CAD build for the part. Positions are in the model's coordinates, mm. Round coordinates to 2 decimals unless told otherwise and drop trailing zeros. One line per question, with ' | ' between items.
```python
from build123d import *

# Parameters (mm, degrees)
SKETCH1_W           = 47.625
SKETCH1_H           = 47.625
SKETCH1_R           = 1.5875
BOSS_EXTRUDE1_DEPTH = 1.5875
FILLET1_R           = 4.7625


with BuildPart() as part:
    # Sketch1 → Boss-Extrude1 (new body)
    with BuildSketch(Plane(origin=(0, 0, 0), x_dir=(1, 0, 0), z_dir=(0, 1, 0))):
        Rectangle(SKETCH1_W, SKETCH1_H)
        with Locations((-19.05, 19.05)):
            Circle(SKETCH1_R, mode=Mode.SUBTRACT)
        with Locations((19.05, 19.05)):
            Circle(SKETCH1_R, mode=Mode.SUBTRACT)
        with Locations((19.05, -19.05)):
            Circle(SKETCH1_R, mode=Mode.SUBTRACT)
        with Locations((-19.05, -19.05)):
            Circle(SKETCH1_R, mode=Mode.SUBTRACT)
    extrude(amount=BOSS_EXTRUDE1_DEPTH)

    # Fillet1
    fillet1_edges = [part.edges().sort_by_distance(p)[0] for p in [
        (-23.8125, 0.79375, -23.8125),
        (23.8125, 0.79375, -23.8125),
        (23.8125, 0.79375, 23.8125),
        (-23.8125, 0.79375, 23.8125),
    ]]
    fillet(fillet1_edges, radius=FILLET1_R)


solid = part.part
```
(1) Two-plate mould, pull along X, no slides. Class faces 1 (the face through (-23.812, 1, 0)), 2 (the face through (-20.22, 0.783, 17.977)), 3 (the face through (0, 1, -23.812)), 4 (the face through (17.88, 0.783, 17.977)): released by +X, released by -X, zero draft, split by the parting line, or undercut.
Results found:
face 1: released by -X | face 2: undercut | face 3: zero draft | face 4: undercut
(2) Probe L1, parallel to Z at x = 19.05, y = 1.15; L2, parallel to Z at x = -21, y = 0.85. List the from-to ranges inside material, lowest first.
Results found:
L1: z = -23.81 to -20.64, -17.46 to 17.46, 20.64 to 23.81 | L2: z = -23.39 to 23.39
(3) Cut at A-A, the plane y = 0.5. State how many separate pieces and enclosed holes the cut face has, then the cut area to 3 significant figures.
Results found:
separate pieces: 1 | enclosed holes: 4 | area: 2,220 mm²
